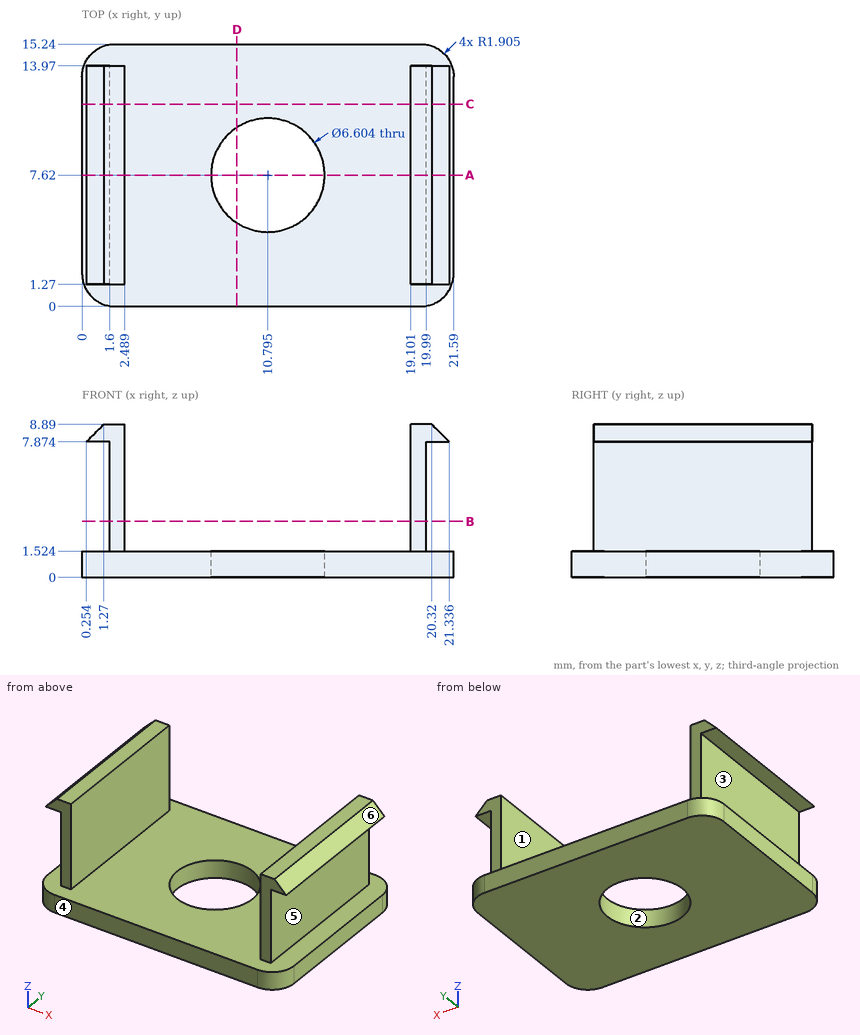
Source: three-view drawing plus pictorial views. Frame: mm from the lowest corner of the part. A direction names the side the tool comes from. Give positions to 0.01 mm unless a question says otherwise; leave off trailing zeros. Order: outer loops, then holes, each group sorted by start corner. A loop starts at its lowest first (then second) coordinate and runs counter-clockwise, first axis right, second up. Notation, with made-up numbers: M 5,83.25 L 50,83.25 A22 cw 50,90.25 Z; hole C 76,24 d6. An arc over 180 degrees is marked long. One line per question, with ' | ' between items.
1) Section A-A on y = 7.62. Output: boundary loops of the cut face in (x, z).
Filled in:
outline: M 0,0 L 7.49,0 L 7.49,1.52 L 2.49,1.52 L 2.49,8.89 L 1.27,8.89 L 0.25,7.87 L 1.6,7.87 L 1.6,1.52 L 0,1.52 Z; M 14.1,0 L 21.59,0 L 21.59,1.52 L 19.99,1.52 L 19.99,7.87 L 21.34,7.87 L 20.32,8.89 L 19.1,8.89 L 19.1,1.52 L 14.1,1.52 Z
2) Section B-B on z = 3.25. Output: boundary loops of the cut face in (x, y).
Filled in:
outline: M 1.6,1.27 L 2.49,1.27 L 2.49,13.97 L 1.6,13.97 Z; M 19.1,1.27 L 19.99,1.27 L 19.99,13.97 L 19.1,13.97 Z
3) Draft query along Z for the marked faces 4, 5 and 6. Return one class per face: pulls with the +Z half, pulls with the -Z half, needs draft (parallel to the pull), parting line crosses it, or undercut.
Filled in:
face 4: needs draft | face 5: undercut | face 6: pulls with the +Z half
4) Section D-D on x = 9. Output: boundary loops of the cut face in (y, z), and give its area (3 significant figures).
Filled in:
outline: M 0,0 L 4.85,0 L 4.85,1.52 L 0,1.52 Z; M 10.39,0 L 15.24,0 L 15.24,1.52 L 10.39,1.52 Z | area: 14.8 mm2
5) Access query for the marked faces 1, 2 and 3. Directions: +Z, -Z, +X, -X, +Y, -Y. A direction counts if a zero-diameter tool reaches every point of the face in a straight line with its end or side. Return the directions, or none.
Filled in:
face 1: +Z, +Y, -Y | face 2: +Z, -Z | face 3: -X, +Y, -Y
6) Ray query, L1, parallel to X at y = 11.5, z = 4.5; L2, parallel to Z at x = 4.5, y = 9; L3, parallel to X at y = 7.75, z = 1.25. Return the intervals inside material, ascending.
Filled in:
L1: x = 1.6 to 2.49, 19.1 to 19.99 | L2: z = 0 to 1.52 | L3: x = 0 to 7.5, 14.09 to 21.59
7) Contact query for flat-ended pins moving along their axis: P1, Ø1, axis at y = 6, z = 6, coming from the +X side; P2, Ø0.7, axis at x = 1, z = 5.5, coming from the -Y side; P3, Ø1.5, axis at x = 1, y = 9, coming from the -Z side; P4, Ø1.8, axis at x = 20.5, z = 7, coming from the -Y side. Output: stop coordinate, or through.
Filled in:
P1: stops at x = 19.99 | P2: passes through | P3: stops at z = 0 | P4: stops at y = 1.27
8) Section C-C on y = 11.75. Output: boundary loops of the cut face in (x, z), and give its area (3 significant figures).
Filled in:
outline: M 0,0 L 21.59,0 L 21.59,1.52 L 19.99,1.52 L 19.99,7.87 L 21.34,7.87 L 20.32,8.89 L 19.1,8.89 L 19.1,1.52 L 2.49,1.52 L 2.49,8.89 L 1.27,8.89 L 0.25,7.87 L 1.6,7.87 L 1.6,1.52 L 0,1.52 Z | area: 47.7 mm2
